```python
from build123d import *

# Parameters (mm, degrees)
F1_DEPTH = 101.6
F3_DEPTH = 76.2
F4_W     = 25.0135893855
F4_H     = 20.0843550265
F5_DEPTH = 103.378
F6_R     = 4.9794966454
F7_DEPTH = 167.132


with BuildPart() as f1:
    # F0 (on Front) → F1 (new body)
    with BuildSketch(Plane.XZ):
        Polygon((-99.4555056095, 23.3819726855), (-99.4555056095, -18.3572731912), (-99.4555056095, -28.7481807172), (-16.8563630432, -28.7481807172), (-16.8563630432, -44.4500036538), (9.9582020193, -44.4500036538), (9.9582020193, 4.0893019177), (-10.5538228527, 23.3819726855), align=None)
    extrude(amount=F1_DEPTH)

    # F2 (on face) → F3 (join)
    with BuildSketch(Plane(origin=(0, 0, 0), x_dir=(-1, 0, 0), z_dir=(0, 1, 0))):
        Polygon((-9.9582020193, -44.4500036538), (-9.9582020193, 4.0893019177), (-61.5653358961, -44.4500036538), align=None)
    extrude(amount=-F3_DEPTH)

    # F4 (on face) → F5 (cut)
    with BuildSketch(Plane(origin=(-99.4555056095, 0, 0), x_dir=(0, -1, 0), z_dir=(-1, 0, 0))):
        with Locations((48.7646157427, 23.3819726855)):
            Rectangle(F4_W, F4_H)
    extrude(amount=-F5_DEPTH, mode=Mode.SUBTRACT)

    # F6 (on face) → F7 (cut)
    with BuildSketch(Plane(origin=(-99.4555056095, 0, 0), x_dir=(0, -1, 0), z_dir=(-1, 0, 0))):
        with Locations((18.2879269123, 0)):
            Circle(F6_R)
        with BuildLine():
            Line((62.3561588025, -28.7481807172), (52.4646214301, -28.7481807172))
            ThreePointArc((52.4646214301, -28.7481807172), (57.4103901163, -33.1490937952), (62.3561588025, -28.7481807172))
        make_face()
        with BuildLine():
            ThreePointArc((62.3898867617, -28.1695971498), (57.1206072149, -23.1985396455), (52.4646214301, -28.7481807172))
            Line((52.4646214301, -28.7481807172), (62.3561588025, -28.7481807172))
            ThreePointArc((62.3561588025, -28.7481807172), (62.3814476206, -28.4593800512), (62.3898867617, -28.1695971498))
        make_face()
        with Locations((58.4661085159, 3.1419980805)):
            Circle(F6_R)
        with BuildLine():
            Line((22.1901210724, -28.7481807172), (12.274295953, -28.7481807172))
            ThreePointArc((12.274295953, -28.7481807172), (17.2322085127, -33.264546828), (22.1901210724, -28.7481807172))
        make_face()
        with BuildLine():
            ThreePointArc((22.1901210724, -28.7481807172), (22.2063062098, -28.5168667938), (22.2117051581, -28.2850501826))
            ThreePointArc((22.2117051581, -28.2850501826), (17.0003919016, -23.3109524855), (12.274295953, -28.7481807172))
            Line((12.274295953, -28.7481807172), (22.1901210724, -28.7481807172))
        make_face()
    extrude(amount=-F7_DEPTH, mode=Mode.SUBTRACT)


solid = f1.part
```
Here's how the part is built. I have some questions about the finished solid (model axes, mm). A direction names the side the tool comes from. Coordinates: 2 decimals unless noted, no trailing zeros. Order: outer loops, then holes, each group sorted by start corner. A loop starts at its lowest first (then second) coordinate and runs counter-clockwise, first axis right, second up. Notation, with made-up numbers: M 84,-3 L 90,-3 A30 ccw 90,31 Z; hole C 38,-13 d6. An arc over 180 degrees is marked long. Answer as a JSON object with one key per item and string values. Group by question number.
(1) For pin 1 (5 mm diameter, centred on y = -47.5, z = -27, fed in from +X); pin 2 (13.5 mm diameter, centred on x = -49.5, y = -9, fed in from -Z); pin 3 (20.5 mm diameter, centred on y = -88.5, z = -26, fed in from +X), each with a flat end and sliding along its axis, tell me the tip position at first contact or that it passes through.
(2) Suppose I cut it at C-C, the plane x = 5. Please give me the cut outline in (y, z), then the cut area to 3 significant figures.
(3) If we mould it in two halves opening along Z, with no side actions, what happens to faces 6 (the face through (-40.76, -17.21, -4.86)), 7 (the face through (-50, -61.271, 18)), 8 (the face through (-54, -81, 23.382))? For each: released by +Z, released by -Z, zero draft, split by the parting line, or undercut.
(4) Suppose I cut it at A-A, the plane z = -31. Please give me the cut outline in (x, y), then the cut area to 3 significant figures.
(5) Suppose I cut it at D-D, the plane x = -80. Please give me the cut outline in (y, z), then the cut area to 3 significant figures.
(6) I need wall thicknesses on probe 1 along Y at (x, z) = (-21, 0); probe 2 along Y at (x, z) = (-23, 13.5); probe 3 along Z at (x, y) = (8.5, -18) (3 decimals). Which ranges of each line are inside material? Lowest first, please.
(7) Suppose I cut it at B-B, the plane y = -57. Please give me the cut outline in (x, z).
(8) Which directions (+Z, -Z, +X, -X, +Y, -Y) give clear straight access to the entire face, cutting with the end or side of a thin tool? Please do faces 1 (the face through (-50, -49, 13.34)), 2 (the face through (-59, -37, -28.748)), 3 (the face through (-36, 0, -10)), 4 (the face through (9.958, -89, -21)), 5 (the face through (-42.408, -60.764, -1.276)).
Values found:
{
 "1": {"pin 1": "stops at x = 45.67", "pin 2": "stops at z = -28.75", "pin 3": "stops at x = 9.96"},
 "2": {"outline": "M -101.6,-44.45 L 0,-44.45 L 0,8.75 L -101.6,8.75 Z; hole C -58.47,3.14 d9.96; hole C -57.41,-28.17 d9.96; hole C -18.29,0 d9.96; hole C -17.23,-28.29 d9.96", "area": "5,090 mm^2"},
 "3": {"face 6": "undercut", "face 7": "zero draft", "face 8": "released by +Z"},
 "4": {"outline": "M -16.86,-101.6 L 9.96,-101.6 L 9.96,-76.2 L 47.27,-76.2 L 47.27,-61.51 L -16.86,-61.51 Z; M -16.86,-53.31 L 47.27,-53.31 L 47.27,-21.41 L -16.86,-21.41 Z; M -16.86,-13.06 L 47.27,-13.06 L 47.27,0 L -16.86,0 Z", "area": "4,510 mm^2"},
 "5": {"outline": "M -101.6,-28.75 L -62.36,-28.75 A4.98 cw long -52.46,-28.75 L -22.19,-28.75 A4.98 cw long -12.27,-28.75 L 0,-28.75 L 0,23.38 L -36.26,23.38 L -36.26,13.34 L -61.27,13.34 L -61.27,23.38 L -101.6,23.38 Z; hole C -58.47,3.14 d9.96; hole C -18.29,0 d9.96", "area": "4,800 mm^2"},
 "6": {"probe 1": "y = -101.6 to -62.33, -54.6 to -23.27, -13.31 to 0", "probe 2": "y = -101.6 to -61.27, -36.26 to 0", "probe 3": "z = -44.45 to -33.205, -23.365 to -4.971, 4.971 to 5.461"},
 "7": {"outline": "M -99.46,-23.21 L 38.98,-23.21 L 16.02,-1.62 L -99.46,-1.62 Z; M -99.46,7.9 L 5.91,7.9 L 0.12,13.34 L -99.46,13.34 Z; M -16.86,-44.45 L 61.57,-44.45 L 49.53,-33.13 L -16.86,-33.13 Z"},
 "8": {"face 1": "+Z, +X, -X", "face 2": "-Z, -X, +Y, -Y", "face 3": "+Z, -Z, +X, -X, +Y", "face 4": "+Z, -Z, +X, -Y", "face 5": "+X, -X"}
}
